The model under review builds one solid part; all positions refer to its coordinate system, in mm. A direction names the side the tool comes from. Coordinates: 2 decimals unless noted, no trailing zeros. Order: outer loops, then holes, each group sorted by start corner. A loop starts at its lowest first (then second) coordinate and runs counter-clockwise, first axis right, second up.
```python
from build123d import *

# Parameters (mm, degrees)
SKETCH1_R           = 3.795
BOSS_EXTRUDE1_DEPTH = 10
BOSS_EXTRUDE2_DEPTH = 180
SKETCH4_R           = 3.795
BOSS_EXTRUDE3_DEPTH = 10
SKETCH7_R           = 3.795
BOSS_EXTRUDE6_DEPTH = 5
SKETCH7_2_R         = 3.795
BOSS_EXTRUDE7_DEPTH = 15
BOSS_EXTRUDE8_DEPTH = 10
SKETCH9_W           = 479.703862309
SKETCH9_H           = 160
CUT_EXTRUDE1_DEPTH  = 11.081066739


with BuildPart() as part:
    # Sketch1 → Boss-Extrude1 (new body, symmetric)
    with BuildSketch(Plane.XY):
        with Locations((354.729090947, 111.880692363)):
            Circle(SKETCH1_R)
    extrude(amount=BOSS_EXTRUDE1_DEPTH, both=True)

    # Sketch3 → Boss-Extrude2 (add)
    with BuildSketch(Plane.XY.offset(10)):
        Polygon((367.212888015, 116.921199692), (342.212888015, 116.840185034), (342.245293879, 106.840185034), (367.245293879, 106.921199692), align=None)
    extrude(amount=BOSS_EXTRUDE2_DEPTH)

    # Sketch4 → Boss-Extrude3 (add)
    with BuildSketch(Plane.XY.offset(190)):
        with Locations((354.729090947, 111.880692363)):
            Circle(SKETCH4_R)
    extrude(amount=BOSS_EXTRUDE3_DEPTH)

    # Sketch7 → Boss-Extrude6 (add)
    with BuildSketch(Plane(origin=(342.587921066, 1.110185725, 0), x_dir=(0, 0, 1), z_dir=(-0.999994749, -0.003240569, 0))):
        with BuildLine():
            Line((10, 115.730606971), (10, 125.730606971))
            ThreePointArc((10, 125.730606971), (20, 135.730606971), (30, 125.730606971))
            Line((30, 125.730606971), (30, 115.730606971))
            Line((30, 115.730606971), (10, 115.730606971))
        make_face()
        with Locations((20, 125.730606971)):
            Circle(SKETCH7_R, mode=Mode.SUBTRACT)
    boss_extrude6 = extrude(amount=-BOSS_EXTRUDE6_DEPTH)

    # Sketch7_2 → Boss-Extrude7 (add)
    with BuildSketch(Plane(origin=(342.587921066, 1.110185725, 0), x_dir=(0, 0, 1), z_dir=(-0.999994749, -0.003240569, 0))):
        with Locations((20, 125.730606971)):
            Circle(SKETCH7_2_R)
    boss_extrude7 = extrude(amount=-BOSS_EXTRUDE7_DEPTH)

    # Mirror2: Boss-Extrude6, Boss-Extrude7 across plane
    add(boss_extrude6.mirror(Plane.XY.offset(100)))
    add(boss_extrude7.mirror(Plane.XY.offset(100)))

    # Sketch8 → Boss-Extrude8 (add)
    with BuildSketch(Plane(origin=(347.587894813, 1.126388571, 0), x_dir=(0, 0, -1), z_dir=(0.999994749, 0.003240569, 0))):
        with BuildLine():
            Line((-180, 131.525606971), (-20, 131.525606971))
            ThreePointArc((-20, 131.525606971), (-14.205, 125.730606971), (-20, 119.935606971))
            Line((-20, 119.935606971), (-180, 119.935606971))
            ThreePointArc((-180, 119.935606971), (-185.795, 125.730606971), (-180, 131.525606971))
        make_face()
        with BuildLine():
            Line((-180, 129.525606971), (-20, 129.525606971))
            ThreePointArc((-20, 129.525606971), (-16.205, 125.730606971), (-20, 121.935606971))
            Line((-20, 121.935606971), (-180, 121.935606971))
            ThreePointArc((-180, 121.935606971), (-183.795, 125.730606971), (-180, 129.525606971))
        make_face(mode=Mode.SUBTRACT)
    extrude(amount=BOSS_EXTRUDE8_DEPTH)

    # Sketch9 → Cut-Extrude1 (cut, through all)
    with BuildSketch(Plane(origin=(-0.375033051, 115.729999309, 0), x_dir=(0.999994749, 0.003240569, 0), z_dir=(-0.003240569, 0.999994749, 0))):
        with Locations((127.73792, -100)):
            Rectangle(SKETCH9_W, SKETCH9_H)
    extrude(amount=-CUT_EXTRUDE1_DEPTH, mode=Mode.SUBTRACT)


solid = part.part
```
(1) For pin 1 Ø5 at (y, z) = (121.5, 25) entering from +X; pin 2 Ø8 at (x, z) = (355.5, 67.5) entering from +Y; pin 3 Ø10 at (x, y) = (349, 128) entering from +Z; pin 4 Ø10 at (x, y) = (354, 116) entering from +Z, all flat-tipped, find the tip position at first contact; note any pin that passes through.
A:
pin 1: stops at x = 357.2
pin 2: stops at y = 132.68
pin 3: stops at z = 190
pin 4: stops at z = 200
(2) We need section C-C, the plane x = 362.75. Write out the cut boundary in (y, z), and give its area (3 significant figures).
A:
outline: (106.91, 10) - (116.91, 10) - (116.91, 20) - (106.91, 20) - close; (106.91, 180) - (116.91, 180) - (116.91, 190) - (106.91, 190) - close
area: 200 mm2
(3) Machinability: for faces 1 (the face through (352.111, 126.789, 23.794)), 2 (the face through (355, 112, 200)), which of the approach directions +Z, -Z, +X, -X, +Y, -Y give a long, thin tool a straight path to every point of the face, cutting with its end or side? Answer none if there is none.
A:
face 1: none
face 2: +Z, +X, -X, +Y, -Y
(4) We need section B-B, the plane y = 110. Write out the cut boundary in (x, z), and give its area (3 significant figures).
A:
outline: (342.24, 10) - (351.43, 10) - (351.43, -10) - (358.03, -10) - (358.03, 10) - (367.24, 10) - (367.24, 20) - (342.24, 20) - close; (342.24, 180) - (367.24, 180) - (367.24, 190) - (358.03, 190) - (358.03, 200) - (351.43, 200) - (351.43, 190) - (342.24, 190) - close
area: 698 mm2
(5) We need section D-D, the plane x = 355. Count the separate pieces of the cut face and the enclosed holes in it, and give its area (3 significant figures).
A:
separate pieces: 3
enclosed holes: 1
area: 1,220 mm2
(6) Wall thickness on probe 1 along Z at (x, y) = (366, 111.5); probe 2 along Y at (x, z) = (348.75, 99); probe 3 along Z at (x, y) = (346.5, 127): over which ranges is each line inside the solid? List them lowest first.
A:
probe 1: z = 10 to 20, 180 to 190
probe 2: y = 121.07 to 123.07, 130.66 to 132.66
probe 3: z = 10 to 30, 170 to 190
(7) We need section A-A, the plane z = 159. Write out the cut boundary in (x, y), and give its area (3 significant figures).
A:
outline: (347.16, 132.65) - (347.17, 130.65) - (357.17, 130.68) - (357.16, 132.68) - close; (347.19, 123.06) - (347.2, 121.06) - (357.2, 121.09) - (357.19, 123.09) - close
area: 40.0 mm2
(8) Draft analysis for pull direction Z (two halves, no side actions). For faces 3 (the face through (355, 112, 20)), 4 (the face through (352.111, 126.745, 185.794)), 5 (the face through (355, 112, -10)), state which applies: released by +Z, released by -Z, zero draft, split by the parting line, or undercut.
A:
face 3: undercut
face 4: released by +Z
face 5: released by -Z
